For this review, take the finished solid that the model builds, in its own axes (mm). A direction names the side the tool comes from. Give positions to 0.01 mm unless a question says otherwise; leave off trailing zeros. Order: outer loops, then holes, each group sorted by start corner. A loop starts at its lowest first (then second) coordinate and runs counter-clockwise, first axis right, second up. Notation, with made-up numbers: (70.5, -31) - (117.5, -31) arc R28 ccw to (117.5, -6) - close; hole circle Ø6 at (-36.75, 9). An arc over 180 degrees is marked (long way). Use a Markdown table: item, result. Add a question column.
1) Mouldability with a two-part tool opening along Z and no side actions: class faces 6 (the face through (-1.8, 1, 2.5)), 7 (the face through (-3.25, 3, 0)), 8 (the face through (0, 3, 4)) as released by +Z, released by -Z, zero draft, split by the parting line, or undercut.
2) Machinability: for faces 1 (the face through (-2.42, 5.4, 0.91)), 2 (the face through (0, 1.2, -4)), 3 (the face through (0, 1.5, -3.5)), 4 (the face through (0, 1, -2)), 5 (the face through (3.25, 3, 0)), which of the approach directions +Z, -Z, +X, -X, +Y, -Y give a long, thin tool a straight path to every point of the face, cutting with its end or side? Answer none if there is none.
3) Wall thickness on L1, parallel to X at y = 0.3, z = 0.75; L2, parallel to Z at x = 0, y = 0.3; L3, parallel to X at y = 3.2, z = -3.5: over which ranges is each line inside the solid? List them lowest first.
4) Clearance check with flat-ended pins moving along their axes: P1, Ø2, axis at y = 4.5, z = 2, coming from the -X side; P2, Ø1, axis at x = -0.5, y = 2.5, coming from the -Z side; P3, Ø0.5, axis at x = -0.5, z = -3.5, coming from the +Y side. State where each tip first meets the part, or that it passes through.
5) We need section A-A on z = -2. Write out the cut boundary in (x, y).
6) We need section C-C on z = -0.5. Write out the cut boundary in (x, y), then the cut area to 3 significant figures.
7) We need section B-B on y = 0.75. Write out the cut boundary in (x, z), then the cut area to 3 significant figures.
8) We need section D-D on x = -0.5. Write out the cut boundary in (y, z), then the cut area to 3 significant figures.
```python
from build123d import *

# Parameters (mm, degrees)
F0_W     = 6.5
F0_H     = 8
F1_DEPTH = 5.4
F2_T     = -1
F3_W     = 3.1
F3_H     = 3.9
F4_DEPTH = 1
F5_W     = 15
F5_H     = 15
F6_DEPTH = 1
F7_R     = 2.25
F8_DEPTH = 25


with BuildPart() as f1:
    # F0 (on Front) → F1 (new body)
    with BuildSketch(Plane.XZ):
        Rectangle(F0_W, F0_H)
    extrude(amount=-F1_DEPTH)

    # F2
    f2_openings = [f1.faces().sort_by_distance(p)[0] for p in [
        (0, 5.4, 0),
    ]]
    offset(amount=F2_T, openings=f2_openings)

    # F3 (on face) → F4 (cut)
    with BuildSketch(Plane(origin=(0, 0, -4), x_dir=(1, 0, 0), z_dir=(0, 0, -1))):
        with Locations((0, -3.45)):
            Rectangle(F3_W, F3_H)
    extrude(amount=-F4_DEPTH, mode=Mode.SUBTRACT)

    # F5 (on face) → F6 (join)
    with BuildSketch(Plane.XZ):
        Rectangle(F5_W, F5_H)
    extrude(amount=-F6_DEPTH)

    # F7 (on face) → F8 (cut)
    with BuildSketch(Plane.XZ):
        with Locations((0, 0.75)):
            Circle(F7_R)
    extrude(amount=-F8_DEPTH, mode=Mode.SUBTRACT)


solid = f1.part
```
Checked values:
| question | item | result |
|---|---|---|
| 1 | face 6 | undercut |
| 1 | face 7 | zero draft |
| 1 | face 8 | released by +Z |
| 2 | face 1 | +Z, -Z, +X, -X, +Y |
| 2 | face 2 | -Z, +X, -X, +Y |
| 2 | face 3 | -Z, +Y |
| 2 | face 4 | +Y |
| 2 | face 5 | +Z, -Z, +X, +Y |
| 3 | L1 | -7.5 to -2.25, 2.25 to 7.5 |
| 3 | L2 | -7.5 to -1.5, 3 to 7.5 |
| 3 | L3 | -3.25 to -1.55, 1.55 to 3.25 |
| 4 | P1 | x = -3.25 |
| 4 | P2 | z = 3 |
| 4 | P3 | y = 1.5 |
| 5 | outline | (-7.5, 0) - (7.5, 0) - (7.5, 1) - (3.25, 1) - (3.25, 5.4) - (2.25, 5.4) - (2.25, 1) - (-2.25, 1) - (-2.25, 5.4) - (-3.25, 5.4) - (-3.25, 1) - (-7.5, 1) - close |
| 6 | outline | (-7.5, 0) - (-1.87, 0) - (-1.87, 1) - (-2.25, 1) - (-2.25, 5.4) - (-3.25, 5.4) - (-3.25, 1) - (-7.5, 1) - close; (1.87, 0) - (7.5, 0) - (7.5, 1) - (3.25, 1) - (3.25, 5.4) - (2.25, 5.4) - (2.25, 1) - (1.87, 1) - close |
| 6 | area | 20.1 mm² |
| 7 | outline | (-7.5, -7.5) - (7.5, -7.5) - (7.5, 7.5) - (-7.5, 7.5) - close; hole circle Ø4.5 at (0, 0.75) |
| 7 | area | 209 mm² |
| 8 | outline | (0, -7.5) - (1, -7.5) - (1, -4) - (1.5, -4) - (1.5, -3) - (1, -3) - (1, -1.44) - (0, -1.44) - close; (0, 2.94) - (1, 2.94) - (1, 3) - (5.4, 3) - (5.4, 4) - (1, 4) - (1, 7.5) - (0, 7.5) - close |
| 8 | area | 15.5 mm² |
